Autodesk Inventor part; units mm, degrees
ref_plane "Work Plane2" through (-24.7933, -29.2153, 105) normal (1, 0, 0) x (0, 1, 0)
ref_plane "YZ Plane" through (0, 0, 0) normal (1, 0, 0) x (0, 1, 0)
ref_plane "XZ Plane" through (0, 0, 0) normal (0, 1, 0) x (-1, 0, 0)
sketch "Sketch1" plane through (0, 0, 0) normal (0, 0, 1) x (1, 0, 0)
  line L0 (-37.5, 35) -> (37.5, 35)
  line L1 (37.5, 35) -> (37.5, -35)
  line L2 (37.5, -35) -> (-37.5, -35)
  line L3 (-37.5, -35) -> (-37.5, 35)
  line L4 (-37.5, 35) -> (37.5, -35) construction
  line L5 (37.5, 35) -> (-37.5, -35) construction
  point P0 (0, 0)
  dimension "d0" = 75
  dimension "d1" = 70
extrude "Extrusion1" add sketch "Sketch1" along normal blind 105
sketch "Sketch2" plane through (0, 0, 105) normal (0, 0, 1) x (1, 0, 0)
  circle A0 centre (-24.7933, -29.2153) radius 1.5
  circle A1 centre (-20.7933, -29.2153) radius 1.5
  point P0 (0, 0)
  dimension "d4" = 3
  dimension "d5" = 3
  dimension "d6" = 4
ref_plane "Work Plane2" through (-24.7933, -29.2153, 105) normal (1, 0, 0) x (0, 1, 0)
sketch "Sketch3" plane through (-24.7933, -29.2153, 105) normal (1, 0, 0) x (0, 1, 0)
  line L0 (0, 0) -> (-8.28, 12.6748) construction
  line L1 (-8.28, 12.6748) -> (-23.4846, 12.6748) construction
  line L2 (-23.4846, 12.6748) -> (-21.9413, -9.551) construction
  spline S0 degree 3 poles (0, 0) (-8.28, 12.6748) (-23.4846, 12.6748) (-21.9413, -9.551) knots 1 1 1 1 2 2 2 2
  point P0 (29.2153, -105)
sweep "Sweep1" add profiles "Sketch2" path "Sketch3" contours A0
pattern_linear "Rectangular Pattern1" count 2 spacing 4 along (1, 0, 0) of "Sweep1"
properties part number "battery_24V"
The model under review builds one solid part; all positions refer to its coordinate system, in mm. Round coordinates to 2 decimals unless told otherwise and drop trailing zeros. Loops run counter-clockwise (first coordinate to the right, second up) from the corner with the lowest first, then second, coordinate; pieces in that order, holes last. Notation, with made-up numbers: (6.25, 59.25) -> (27.25, 59.25) arc R25 cw to (27.25, 94.25) -> close; hole circle Ø6 at (77.5, 29.25). An arc over 180 degrees is marked (long way). Answer as a JSON object with one key per item and string values. Group by question number.
1) We need section A-A on x = 8. Write out the cut boundary in (y, z).
2) For pin 1 Ø4 at (x, y) = (-24.5, -24.5) entering from +Z; pin 2 Ø12 at (x, z) = (-22, 46.5) entering from -Y; pin 3 Ø2 at (x, y) = (4.5, -10) entering from -Z, all flat-tipped, find the tip position at first contact; note any pin that passes through.
3) We need section B-B on z = 29. Write out the cut boundary in (x, y).
4) For line 1 (Y direction, x = 4, z = 57); line 2 (Z direction, x = 24.5, y = -33.5); line 3 (Z direction, x = -24.5, y = -48), list the stretches that pass through material, from the lowest coordinate up. Write a range as [from, to].
Result set:
{
 "1": {"outline": "(-35, 0) -> (35, 0) -> (35, 105) -> (-35, 105) -> close"},
 "2": {"pin 1": "z = 105", "pin 2": "y = -35", "pin 3": "z = 0"},
 "3": {"outline": "(-37.5, -35) -> (37.5, -35) -> (37.5, 35) -> (-37.5, 35) -> close"},
 "4": {"line 1": "[-35, 35]", "line 2": "[0, 105]", "line 3": "[108.49, 112.45]"}
}
